CAD build for the part. Positions are in the model's coordinates, mm. A direction names the side the tool comes from. Coordinates: 2 decimals unless noted, no trailing zeros. Loops run counter-clockwise (first coordinate to the right, second up) from the corner with the lowest first, then second, coordinate; pieces in that order, holes last. Notation, with made-up numbers: (52.5, 61.5) - (70.5, 61.5) arc R19 ccw to (70.5, 89.5) - close; hole circle Ø3 at (55.25, 78). An arc over 180 degrees is marked (long way). Put each result on its own line as item: value.
```python
from build123d import *

# Parameters (mm, degrees)
SKETCH_1_R               = 2.5
EXTRUDE_1_DEPTH          = 88.2
SKETCH_2_R               = 12.5
EXTRUDE_2_DEPTH          = 62
SKETCH_3_W               = 40
SKETCH_3_H               = 17.730441408
SKETCH_3_R               = 5
EXTRUDE_3_DEPTH          = 3
PATTERN_LINEAR_1_COUNT   = 2
PATTERN_LINEAR_1_PITCH   = 59
CUT_EXTRUDE_1_DEPTH      = 85.347436238
CUT_EXTRUDE_1_DEPTH_BACK = 85.347436238
SKETCH_6_W               = 31.187630179
SKETCH_6_H               = 17.730441408
CUT_EXTRUDE_7_DEPTH      = 6
PATTERN_LINEAR_3_COUNT   = 2
PATTERN_LINEAR_3_PITCH   = 59
CUT_EXTRUDE_8_DEPTH      = 92.595344354
SKETCH_10_W              = 11.2
SKETCH_10_H              = 5
CUT_EXTRUDE_9_DEPTH      = 78.257408107
SKETCH_11_R              = 2.5
CUT_EXTRUDE_10_DEPTH     = 65.470923679


with BuildPart() as part:
    # 草图1 → 凸台-拉伸1 (new body)
    with BuildSketch(Plane.XY):
        Circle(SKETCH_1_R)
    extrude(amount=EXTRUDE_1_DEPTH)

    # 草图2 → 凸台-拉伸2 (add)
    with BuildSketch(Plane.XY.offset(73.2)):
        Circle(SKETCH_2_R)
    extrude(amount=-EXTRUDE_2_DEPTH)

    # 草图3 → 凸台-拉伸3 (add)
    with BuildSketch(Plane.XY.offset(73.2)):
        with Locations((20, 0)):
            Rectangle(SKETCH_3_W, SKETCH_3_H)
        with Locations((32.640039451, 0)):
            Circle(SKETCH_3_R, mode=Mode.SUBTRACT)
    extrude_3 = extrude(amount=-EXTRUDE_3_DEPTH)

    # 阵列(线性)1: 凸台-拉伸3 ×2
    with Locations(*[(0, 0, -i * PATTERN_LINEAR_1_PITCH) for i in range(1, PATTERN_LINEAR_1_COUNT)]):
        add(extrude_3)

    # 草图6 → 切除-拉伸1 (cut, two sides: drawn at the far end of the back side and taken through both)
    with BuildSketch(Plane.XY.offset(73.2).offset(-CUT_EXTRUDE_1_DEPTH_BACK)):
        with Locations((24.406184911, 0)):
            Rectangle(SKETCH_6_W, SKETCH_6_H)
    extrude(amount=CUT_EXTRUDE_1_DEPTH + CUT_EXTRUDE_1_DEPTH_BACK, mode=Mode.SUBTRACT)

    # 草图8 → 切除-拉伸7 (cut)
    with BuildSketch(Plane(origin=(8.812369821, 0, 0), x_dir=(0, 0, -1), z_dir=(1, 0, 0))):
        Polygon((-70.2, 8.865220704), (-72.620989075, 8.865220704), (-73.2, 8.865220704), (-73.2, 6.367777059), (-73.2, -8.865220704), (-70.2, -8.865220704), align=None)
    cut_extrude_7 = extrude(amount=-CUT_EXTRUDE_7_DEPTH, mode=Mode.SUBTRACT)

    # 阵列(线性)3: 切除-拉伸7 ×2
    with Locations(*[(0, 0, -i * PATTERN_LINEAR_3_PITCH) for i in range(1, PATTERN_LINEAR_3_COUNT)]):
        add(cut_extrude_7, mode=Mode.SUBTRACT)

    # 草图9 → 切除-拉伸8 (cut, through all)
    with BuildSketch(Plane(origin=(8.812369821, 0, 0), x_dir=(0, 0, -1), z_dir=(1, 0, 0))):
        Polygon((-73.2, -2.531338833), (-73.2, 2.528560393), (-88.2, 2.5), (-88.2, -2.5), align=None)
    extrude(amount=-CUT_EXTRUDE_8_DEPTH, mode=Mode.SUBTRACT)

    # 草图10 → 切除-拉伸9 (cut, through all)
    with BuildSketch(Plane(origin=(8.812369821, 0, 0), x_dir=(0, 0, -1), z_dir=(1, 0, 0))):
        with Locations((-5.6, 0)):
            Rectangle(SKETCH_10_W, SKETCH_10_H)
    extrude(amount=-CUT_EXTRUDE_9_DEPTH, mode=Mode.SUBTRACT)

    # 草图11 → 切除-拉伸10 (cut, through all)
    with BuildSketch(Plane.XY.offset(73.2)):
        Circle(SKETCH_11_R)
    extrude(amount=-CUT_EXTRUDE_10_DEPTH, mode=Mode.SUBTRACT)


solid = part.part
```
Q1. Slice it at D-D, the plane x = 5.5. Give the cut face in (y, z), then the cut area to 3 significant figures.
Determined:
outline: (-11.22, 11.2) - (-8.87, 11.2) - (-8.87, 14.2) - (8.87, 14.2) - (8.87, 11.2) - (11.22, 11.2) - (11.22, 73.2) - (8.87, 73.2) - (8.87, 70.2) - (-8.87, 70.2) - (-8.87, 73.2) - (-11.22, 73.2) - close
area: 1,290 mm2
Q2. Slice it at B-B, the plane y = 0. Give the cut face in (x, z), then the cut area to 3 significant figures.
Determined:
outline: (-12.5, 11.2) - (-2.5, 11.2) - (-2.5, 73.2) - (-12.5, 73.2) - close; (2.5, 11.2) - (2.81, 11.2) - (2.81, 14.2) - (8.81, 14.2) - (8.81, 70.2) - (2.81, 70.2) - (2.81, 73.2) - (2.5, 73.2) - close
area: 975 mm2
Q3. Mould opens along Y. For faces 1 (the cylindrical face through (-12.493, 0.412, 42.634)), 2 (the flat face through (6, 8.865, 72)), 3 (the flat face through (8.812, 0, 42)) say: +Y half, -Y half, draft (parallel to the pull), parting line (faces both ways), or undercut.
Determined:
face 1: parting line
face 2: undercut
face 3: draft
Q4. Tool access for faces 4 (the flat face through (6, -8.865, 72)), 5 (the cylindrical face through (-0.54, -2.44, 42.63)), 6 (the flat face through (2.812, 0, 13)): list every direction of +Z, -Z, +X, -X, +Y, -Y with a clear straight run to the whole face (end or side of a thin tool).
Determined:
face 4: +Z, +X
face 5: +Z, -Z
face 6: -Z, +X
Q5. Pin check, flat tips, straight feed: pin 1 Ø4 at (y, z) = (-7.5, 43.5) entering from -X (3 decimals); pin 2 Ø5 at (y, z) = (5.5, 52) entering from -X; pin 3 Ø2 at (x, z) = (5, 29) entering from +Y. Stop position of each tip, or through.
Determined:
pin 1: x = -11.225
pin 2: x = -12.13
pin 3: y = 11.84
Q6. Slice it at C-C, the plane z = 27. Give the cut face in (x, y), then the cut area to 3 significant figures.
Determined:
outline: (8.81, -8.87) - (8.81, 8.87) arc R12.5 ccw (long way) to start; hole circle Ø5 at (0, 0)
area: 426 mm2
Q7. Wall check: L1, parallel to Y at x = 0, z = 38; L2, parallel to Z at x = 6.5, y = 0.25; L3, parallel to Y at x = 1.5, z = 40.5. Give the ranges that are in metal, low to high. Write a range as from..to.
Determined:
L1: -12.5..-2.5, 2.5..12.5
L2: 14.2..70.2
L3: -12.41..-2, 2..12.41
Q8. Slice it at A-A, the plane x = 0. Give the cut face in (y, z).
Determined:
outline: (-12.5, 11.2) - (-2.5, 11.2) - (-2.5, 73.2) - (-12.5, 73.2) - close; (2.5, 11.2) - (12.5, 11.2) - (12.5, 73.2) - (2.5, 73.2) - close
